Source: CAD feature listing. Evaluate the final solid. Frame: model axes, mm. A direction names the side the tool comes from. Give positions to 0.01 mm unless a question says otherwise; leave off trailing zeros. Order: outer loops, then holes, each group sorted by start corner. A loop starts at its lowest first (then second) coordinate and runs counter-clockwise, first axis right, second up.
1) Material intervals for line 1 (Y direction, x = -11.5, z = 1.45); line 2 (X direction, y = -3.5, z = 1.35) (3 decimals); line 3 (X direction, y = 11.5, z = 0.6), sorted ascending.
2) Access query for faces 1 (the face through (0, -9.42, 1)), 2 (the face through (0, -1, 0)), 3 (the face through (20.52, 2, 1)). Directions: +Z, -Z, +X, -X, +Y, -Y. A direction counts if a zero-diameter tool reaches every point of the face in a straight line with its end or side. Return the directions, or none.
3) Section B-B, the plane y = -7.5. Return loops of the section in (x, z), plus the area to 3 significant figures.
4) Section D-D, the plane y = -3. Return loops of the section in (x, z) (3 decimals).
5) Section A-A, the plane x = -15. Return loops of the section in (y, z), plus the area to 3 significant figures.
6) Draft query along X for faces 4 (the face through (0, -19, 0.3)), 5 (the face through (0, 2, 1.3)), 6 (the face through (-20.52, 2, 1)). Return one class per face: released by +X, released by -X, zero draft, split by the parting line, or undercut.
7) Section C-C, the plane z = 0.9. Return loops of the section in (x, y), plus the area to 3 significant figures.
8) First-contact query: P1, Ø11, axis at x = 2, y = -17, coming from the +Z side; P2, Ø2, axis at x = 11, y = -15.5, coming from the -Z side; P3, Ø8, axis at x = -14, y = -9.5, coming from the -Z side; P4, Ø5.5, axis at x = -6.5, y = -0.5, coming from the +Z side. Flat tips, straight axial feed; report the tip coordinate or a pass-through.
Solid Edge part; units mm, degrees
sketch "Sketch1" plane through (0, 0, 0) normal (0, 0, 1) x (1, 0, 0)
  line L0 (-21.02, -13.61) -> (21.02, -13.61)
  line L1 (21.02, -13.61) -> (21.02, 13.61)
  line L2 (21.02, 13.61) -> (-21.02, 13.61)
  line L3 (-21.02, 13.61) -> (-21.02, -13.61)
  dimension "D1" = 21.02
  dimension "D2" = 21.02
extrude "Protrusion1" add sketch "Sketch1" along normal blind 0.5
sketch "Sketch2" plane through (0, 0, 0.5) normal (0, 0, 1) x (1, 0, 0)
  line L0 (-20.52, -9.42) -> (20.52, -9.42)
  line L1 (20.52, -9.42) -> (20.52, 13.61)
  line L2 (20.52, 13.61) -> (-20.52, 13.61)
  line L3 (-20.52, 13.61) -> (-20.52, -9.42)
  dimension "D1" = 20.52
  dimension "D2" = 20.52
extrude "Ausprägung_2" add sketch "Sketch2" along normal blind 1
sketch "Sketch3" plane through (0, 2.095, 1.5) normal (0, 0, 1) x (1, 0, 0)
  line L0 (-17.525, -8.995) -> (17.525, -8.995)
  line L1 (17.525, -8.995) -> (17.525, 8.515)
  line L2 (17.525, 8.515) -> (-17.525, 8.515)
  line L3 (-17.525, 8.515) -> (-17.525, -8.995)
  dimension "D1" = 17.525
  dimension "D2" = 17.525
extrude "Ausschnitt_1" cut sketch "Sketch3" against normal blind 0.2
sketch "Sketch4" plane through (0, 0, 0) normal (0, 0, 1) x (1, 0, 0)
  line L0 (-6.25, -13.61) -> (6.25, -13.61)
  line L1 (6.25, -23.61) -> (6.25, -13.61)
  line L2 (-6.25, -23.61) -> (6.25, -23.61)
  line L3 (-6.25, -13.61) -> (-6.25, -23.61)
  dimension "D1" = 6.25
  dimension "D2" = 6.25
extrude "Ausprägung_3" add sketch "Sketch4" along normal blind 0.3
From the geometry:
1. line 1: y = -9.42 to -6.9, 10.61 to 13.61
1. line 2: x = -20.52 to -17.525, 17.525 to 20.52
1. line 3: x = -20.52 to 20.52
2. face 1: +Z, +X, -X, -Y
2. face 2: -Z, +X, -X, +Y, -Y
2. face 3: +Z, +X, +Y, -Y
3. outline: (-21.02, 0) - (21.02, 0) - (21.02, 0.5) - (20.52, 0.5) - (20.52, 1.5) - (-20.52, 1.5) - (-20.52, 0.5) - (-21.02, 0.5) - close
3. area: 62.1 mm2
4. outline: (-21.02, 0) - (21.02, 0) - (21.02, 0.5) - (20.52, 0.5) - (20.52, 1.5) - (17.525, 1.5) - (17.525, 1.3) - (-17.525, 1.3) - (-17.525, 1.5) - (-20.52, 1.5) - (-20.52, 0.5) - (-21.02, 0.5) - close
5. outline: (-13.61, 0) - (13.61, 0) - (13.61, 1.5) - (10.61, 1.5) - (10.61, 1.3) - (-6.9, 1.3) - (-6.9, 1.5) - (-9.42, 1.5) - (-9.42, 0.5) - (-13.61, 0.5) - close
5. area: 33.1 mm2
6. face 4: zero draft
6. face 5: undercut
6. face 6: released by -X
7. outline: (-20.52, -9.42) - (20.52, -9.42) - (20.52, 13.61) - (-20.52, 13.61) - close
7. area: 945 mm2
8. P1: stops at z = 0.5
8. P2: passes through
8. P3: stops at z = 0
8. P4: stops at z = 1.3
